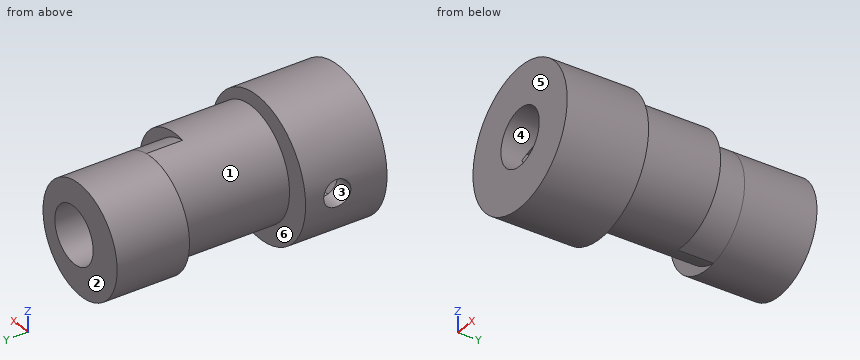
```python
from build123d import *

# Parameters (mm, degrees)
SKETCH1_R           = 7.75
BOSS_EXTRUDE1_DEPTH = 9
SKETCH2_R           = 6.1
BOSS_EXTRUDE2_DEPTH = 12.4
SKETCH4_R           = 6.1
BOSS_EXTRUDE4_DEPTH = 8
SKETCH5_R           = 3.15
CUT_EXTRUDE1_DEPTH  = 32.376503948
SKETCH8_R           = 1.5
CUT_EXTRUDE3_DEPTH  = 32.376503948
SKETCH10_R          = 1.5
CUT_EXTRUDE4_DEPTH  = 5.5
CUT_EXTRUDE5_START  = -4
CUT_EXTRUDE5_DEPTH  = 4


with BuildPart() as part:
    # Sketch1 → Boss-Extrude1 (new body)
    with BuildSketch(Plane(origin=(0, 0, 0), x_dir=(1, 0, 0), z_dir=(0, 1, 0))):
        with Locations(Location((0, 0, 0), (0, 0, 270))):
            Circle(SKETCH1_R)
    extrude(amount=BOSS_EXTRUDE1_DEPTH)

    # Sketch2 → Boss-Extrude2 (add)
    with BuildSketch(Plane(origin=(0, 9, 0), x_dir=(1, 0, 0), z_dir=(0, 1, 0))):
        with Locations(Location((1, 0, 0), (0, 0, 90))):
            Circle(SKETCH2_R)
    extrude(amount=BOSS_EXTRUDE2_DEPTH)

    # Sketch4 → Boss-Extrude4 (add)
    with BuildSketch(Plane(origin=(0, 21.4, 0), x_dir=(1, 0, 0), z_dir=(0, 1, 0))):
        with Locations(Location((-1, 0, 0), (0, 0, 80.564661277))):
            Circle(SKETCH4_R)
    extrude(amount=BOSS_EXTRUDE4_DEPTH)

    # Sketch5 → Cut-Extrude1 (cut, through all)
    with BuildSketch(Plane.XZ):
        with Locations(Location((0, 0, 0), (0, 0, 270))):
            Circle(SKETCH5_R)
    extrude(amount=-CUT_EXTRUDE1_DEPTH, mode=Mode.SUBTRACT)

    # Sketch8 → Cut-Extrude3 (cut, through all)
    with BuildSketch(Plane(origin=(0, 0, 0), x_dir=(0, 0, -1), z_dir=(1, 0, 0))):
        with Locations((0, 5.5)):
            Circle(SKETCH8_R)
    extrude(amount=-CUT_EXTRUDE3_DEPTH, mode=Mode.SUBTRACT)

    # Sketch10 → Cut-Extrude4 (cut)
    with BuildSketch(Plane(origin=(0, 0, 0), x_dir=(0, 0, -1), z_dir=(1, 0, 0))):
        Polygon((0, 8.675426481), (-2.75, 7.08771324), (-2.75, 3.91228676), (0, 2.324573519), (2.75, 3.91228676), (2.75, 7.08771324), align=None)
        with Locations((0, 5.5)):
            Circle(SKETCH10_R, mode=Mode.SUBTRACT)
    extrude(amount=-CUT_EXTRUDE4_DEPTH, mode=Mode.SUBTRACT)

    # Sketch11 → Cut-Extrude5 (cut)
    with BuildSketch(Plane(origin=(0, 21.4, 0), x_dir=(1, 0, 0), z_dir=(0, 1, 0)).offset(CUT_EXTRUDE5_START)):
        with BuildLine():
            ThreePointArc((0, -6.017474553), (5.1, 0), (0, 6.017474553))
            ThreePointArc((0, 6.017474553), (7.1, 0), (0, -6.017474553))
        make_face()
    extrude(amount=CUT_EXTRUDE5_DEPTH, mode=Mode.SUBTRACT)


solid = part.part
```
Source: CAD feature listing. Evaluate the final solid. Frame: model axes, mm. Face numbers are marked on the shaded views. A direction names the side the tool comes from. Round coordinates to 2 decimals unless told otherwise and drop trailing zeros. Loops run counter-clockwise (first coordinate to the right, second up) from the corner with the lowest first, then second, coordinate; pieces in that order, holes last.
1. Ray query, L1, parallel to X at y = 14, z = 0; L2, parallel to Y at x = -1.75, z = 6; L3, parallel to Y at x = 3.75, z = 4. Return the intervals inside material, ascending.
2. Section query B-B on y = 15.25. Output: boundary loops of the cut face in (x, z).
3. Mould query, pull axis Z, two halves, no side actions, for the marked faces 1, 2, 3 and 4. Classes: released by +Z, released by -Z, zero draft, split by the parting line, or undercut.
4. Section query C-C on z = 1. Output: boundary loops of the cut face in (x, y), and give its area (3 significant figures).
5. Section query D-D on x = 6.25. Output: boundary loops of the cut face in (y, z).
6. Access query for the marked faces 5 and 6. Directions: +Z, -Z, +X, -X, +Y, -Y. A direction counts if a zero-diameter tool reaches every point of the face in a straight line with its end or side. Return the directions, or none.
7. Section query A-A on x = 2.5. Output: boundary loops of the cut face in (y, z).
8. Contact query for flat-ended pins moving along their axis: pin 1 (5.5 mm diameter, centred on x = -5, z = -2.5, fed in from -Y); pin 2 (4 mm diameter, centred on x = -2.5, y = 13.5, fed in from -Z); pin 3 (1 mm diameter, centred on x = -3, y = 5.5, fed in from -Z); pin 4 (1.5 mm diameter, centred on y = 24.5, z = 6, fed in from +X). Output: stop coordinate, or through.
Answers below:
1. L1: x = -5.1 to -3.15, 3.15 to 7.1
1. L2: y = 0 to 9, 21.4 to 29.4
1. L3: y = 0 to 17.4
2. outline: circle Ø12.2 at (1, 0); hole circle Ø6.3 at (0, 0)
3. face 1: split by the parting line
3. face 2: zero draft
3. face 3: undercut
3. face 4: undercut
4. outline: (-7.69, 0) - (-2.99, 0) - (-2.99, 2.9) - (-5.5, 2.9) - (-5.5, 4.38) - (-7.69, 4.38) - close; (-7.69, 6.62) - (-5.5, 6.62) - (-5.5, 8.1) - (-2.99, 8.1) - (-2.99, 29.4) - (-7.02, 29.4) - (-7.02, 21.4) - (-5.02, 21.4) - (-5.02, 9) - (-7.69, 9) - close; (2.99, 0) - (7.69, 0) - (7.69, 9) - (7.02, 9) - (7.02, 17.4) - (5.02, 17.4) - (5.02, 29.4) - (2.99, 29.4) - close
4. area: 182 mm2
5. outline: (0, -4.58) - (9, -4.58) - (9, -3.11) - (17.4, -3.11) - (17.4, 3.11) - (9, 3.11) - (9, 4.58) - (0, 4.58) - close
6. face 5: +Z, -Z, +X, -X, -Y
6. face 6: none
7. outline: (0, -7.34) - (9, -7.34) - (9, -5.91) - (17.4, -5.91) - (17.4, -5) - (29.4, -5) - (29.4, -1.92) - (0, -1.92) - close; (0, 1.92) - (29.4, 1.92) - (29.4, 5) - (17.4, 5) - (17.4, 5.91) - (9, 5.91) - (9, 7.34) - (0, 7.34) - close
8. pin 1: stops at y = 0
8. pin 2: stops at z = -5.91
8. pin 3: stops at z = -7.34
8. pin 4: stops at x = 2.11
